from build123d import *

# Parameters (mm, degrees)
SKETCH2_W                    = 40
SKETCH2_H                    = 761
BASE_FLANGE1_DEPTH           = 2
EDGE_FLANGE1_STRIP_W         = 12
EDGE_FLANGE1_STRIP_H         = 2
EDGE_FLANGE1_STRIP_CUT_DEPTH = 761
EDGE_FLANGE1_DEPTH           = 761
FILLET1_R                    = 15
F_7_0_7_DIAMETER_HOLE1_D     = 7


# Sheet-metal steps are written as plain solids
with BuildPart() as part:
    # Sketch2 → Base-Flange1 (new body)
    with BuildSketch(Plane.XY):
        Rectangle(SKETCH2_W, SKETCH2_H)
    extrude(amount=-BASE_FLANGE1_DEPTH)

    # Edge-Flange1 strip (across the edge) → Edge-Flange1 strip cut (cut)
    with BuildSketch(Plane(origin=(20, -380.5, 0), x_dir=(-1, 0, 0), z_dir=(0, 1, 0))):
        with Locations((-2, -1)):
            Rectangle(EDGE_FLANGE1_STRIP_W, EDGE_FLANGE1_STRIP_H)
    extrude(amount=EDGE_FLANGE1_STRIP_CUT_DEPTH, mode=Mode.SUBTRACT)

    # Edge-Flange1 section (across the edge) → Edge-Flange1 (add)
    with BuildSketch(Plane(origin=(20, -380.5, 0), x_dir=(-1, 0, 0), z_dir=(0, 1, 0))):
        with BuildLine():
            Line((0, 2), (0, 20))
            Line((0, 20), (2, 20))
            Line((2, 20), (2, 2))
            ThreePointArc((2, 2), (2.585786438, 0.585786438), (4, 0))
            Line((4, 0), (4, -2))
            ThreePointArc((4, -2), (1.171572875, -0.828427125), (0, 2))
        make_face()
    extrude(amount=EDGE_FLANGE1_DEPTH)

    # Fillet1
    fillet1_edges = [part.edges().sort_by_distance(p)[0] for p in [
        (19, -380.5, 20),
        (19, 380.5, 20),
        (-20, -380.5, -1),
        (-20, 380.5, -1),
    ]]
    fillet(fillet1_edges, radius=FILLET1_R)

    # Ø7.0 (7) Diameter Hole1 (through all)
    with Locations(Plane.XY):
        with Locations((0, 362.5), (0, 181.25), (0, 0), (0, -181.25), (0, -362.5)):
            Hole(F_7_0_7_DIAMETER_HOLE1_D / 2)


solid = part.part
Geometry: final body of the model. Coordinates: model frame, mm. A direction names the side the tool comes from. Give positions to 0.01 mm unless a question says otherwise; leave off trailing zeros. Write each loop counter-clockwise with the first axis right and the second up, starting at its lowest first coordinate (ties: lowest second). Pieces come first, ordered by that corner, then holes. Notation, with made-up numbers: (25.25, 53.5) -> (46.25, 53.5) arc R18 ccw to (46.25, 65.5) -> close; hole circle Ø7 at (41, 66). An arc over 180 degrees is marked (long way). Answer in a Markdown table with one row per item.
(1) Set-up query: faces 1 (the flat face through (18, -5, 11)), 2 (the flat face through (20, -5, 11)). Return all of +Z, -Z, +X, -X, +Y, -Y with unobstructed straight access to the full face (end or side cutting, diameter ignored); none if empty.
Answers below:
| item | result |
|---|---|
| face 1 | +Z, -X, +Y, -Y |
| face 2 | +Z, -Z, +X, +Y, -Y |
(2) Pin query (flat end, axial travel): pin 1 (2 mm diameter, centred on y = 170.5, z = 7, fed in from -X); pin 2 (11 mm diameter, centred on x = 0, y = 0, fed in from +Z). Return the tip coordinate at first contact, or that it passes through.
Answers below:
| item | result |
|---|---|
| pin 1 | x = 18 |
| pin 2 | z = 0 |
(3) Ray query, line 1 along Y through (x, z) = (0, -0.9); line 2 along X through (y, z) = (-181.25, -1.5); line 3 along Z through (x, y) = (-1, 191.5). Return the intervals inside material, ascending. Write a range as [from, to].
Answers below:
| item | result |
|---|---|
| line 1 | [-380.5, -366], [-359, -184.75], [-177.75, -3.5], [3.5, 177.75], [184.75, 359], [366, 380.5] |
| line 2 | [-20, -3.5], [3.5, 17.94] |
| line 3 | [-2, 0] |
(4) Draft query along Y for faces 3 (the cylindrical face through (-15.49, 376.22, -1.01)), 4 (the flat face through (-2, 5, -2)), 5 (the cylindrical face through (18.99, -375.99, 15.72)). Return one class per face: +Y half, -Y half, draft (parallel to the pull), parting line (faces both ways), or undercut.
Answers below:
| item | result |
|---|---|
| face 3 | +Y half |
| face 4 | draft |
| face 5 | -Y half |
(5) Section query A-A on y = -256.5. Return loops of the section in (x, z), then the cut area to 3 significant figures.
Answers below:
| item | result |
|---|---|
| outline | (-20, -2) -> (16, -2) arc R4 ccw to (20, 2) -> (20, 20) -> (18, 20) -> (18, 2) arc R2 cw to (16, 0) -> (-20, 0) -> close |
| area | 117 mm^2 |
(6) Section query B-B on z = 13.75. Return loops of the section in (x, y).
Answers below:
| item | result |
|---|---|
| outline | (18, -377.68) -> (20, -377.68) -> (20, 377.68) -> (18, 377.68) -> close |
